Design review of the part built by this model. Coordinates are the model's own, in mm. A direction names the side the tool comes from. Give positions to 0.01 mm unless a question says otherwise; leave off trailing zeros. Order: outer loops, then holes, each group sorted by start corner. A loop starts at its lowest first (then second) coordinate and runs counter-clockwise, first axis right, second up.
Autodesk Inventor part; units mm, degrees
ref_plane "YZ Plane" through (0, 0, 0) normal (1, 0, 0) x (0, 1, 0)
ref_plane "XZ Plane" through (0, 0, 0) normal (0, 1, 0) x (-1, 0, 0)
ref_plane "XY Plane" through (0, 0, 0) normal (0, 0, 1) x (1, 0, 0)
sketch "Sketch1" plane through (0, 0, 0) normal (0, 0, 1) x (1, 0, 0)
  line L0 (36.9289, 8.8897) -> (11.5289, 8.8897)
  line L1 (36.9289, 148.5897) -> (36.9289, 8.8897)
  line L2 (11.5289, 148.5897) -> (36.9289, 148.5897)
  line L3 (20.8517, 15.2397) -> (20.8517, 142.2397)
  arc A0 (27.6081, 142.2397) -> (20.8517, 142.2397) centre (24.2299, 142.2397) ccw
  line L4 (27.6081, 142.2397) -> (27.6081, 15.2397)
  arc A1 (20.8517, 15.2397) -> (27.6081, 15.2397) centre (24.2299, 15.2397) ccw
  line L5 (36.9289, 148.5897) -> (11.5289, 148.5897)
  line L6 (11.5289, 148.5897) -> (11.5289, 8.8897)
  point P0 (0, 0)
  point P1 (0, 0)
  dimension "d0" = 25.4
  dimension "d2" = 139.7
  dimension "d5" = 6.35
  dimension "d6" = 6.35
  dimension "d7" = 3.3782
  dimension "d8" = 6.7564
  dimension "d9" = 3.3782
extrude "Plate1" add sketch "Sketch1" along normal blind 3.175
fillet "Corner Round1" radius 6.35 4 edges at (36.9289, 148.5897, 1.5875) (11.5289, 148.5897, 1.5875) (36.9289, 8.8897, 1.5875) (11.5289, 8.8897, 1.5875)
equation "\"BendRadius\" = Thickness"
equation "\"BendReliefWidth\" = Thickness"
equation "\"BendReliefDepth\" = 0.5 * Thickness"
equation "\"CornerReliefSize\" = 4 * Thickness"
equation "\"MinimumRemnant\" = 2 * Thickness"
equation "\"TransitionRadius\" = BendRadius"
equation "\"JacobiRadiusSize\" = BendRadius"
equation "\"GapSize\" = Thickness"
equation "\"d1\" = BendRadius"
properties part number "back brace mount" material "Aluminum 6061"
1. Machinability: for faces 4 (the face through (20.852, 78, 2)), 5 (the face through (35.02, 10.7, 1.61)), which of the approach directions +Z, -Z, +X, -X, +Y, -Y give a long, thin tool a straight path to every point of the face, cutting with its end or side? Answer none if there is none.
Recorded:
face 4: +Z, -Z
face 5: +Z, -Z, +X, -Y
2. Take a section at B-B (x = 25.5). State the section outline as (y, z) points (3 decimals), then the cut area to 3 significant figures.
Recorded:
outline: (8.89, 0) - (12.109, 0) - (12.109, 3.175) - (8.89, 3.175) - close; (145.37, 0) - (148.59, 0) - (148.59, 3.175) - (145.37, 3.175) - close
area: 20.4 mm2
3. Take a section at C-C (z = 2.5). State the section outline as (x, y) points, then the cut area to 3 significant figures.
Recorded:
outline: (11.53, 15.24) arc R6.35 ccw to (17.88, 8.89) - (30.58, 8.89) arc R6.35 ccw to (36.93, 15.24) - (36.93, 142.24) arc R6.35 ccw to (30.58, 148.59) - (17.88, 148.59) arc R6.35 ccw to (11.53, 142.24) - close; hole (20.85, 15.24) arc R3.38 ccw to (27.61, 15.24) - (27.61, 142.24) arc R3.38 ccw to (20.85, 142.24) - close
area: 2,620 mm2
4. Draft analysis for pull direction Y (two halves, no side actions). For faces 1 (the face through (30, 80, 3.175)), 2 (the face through (35.1, 146.7, 1.6)), 3 (the face through (24.304, 11.862, 1.565)), state which applies: pulls with the +Y half, pulls with the -Y half, needs draft (parallel to the pull), parting line crosses it, or undercut.
Recorded:
face 1: needs draft
face 2: pulls with the +Y half
face 3: undercut
5. For pin 1 (1 mm diameter, centred on x = 16.5, z = 1, fed in from +Y); pin 2 (2 mm diameter, centred on x = 23.5, y = 86, fed in from -Z), all flat-tipped, find the tip position at first contact; note any pin that passes through.
Recorded:
pin 1: stops at y = 148.53
pin 2: passes through
6. Take a section at A-A (y = 124.5). State the section outline as (x, z) points (3 decimals), then the cut area to 3 significant figures.
Recorded:
outline: (11.529, 0) - (20.852, 0) - (20.852, 3.175) - (11.529, 3.175) - close; (27.608, 0) - (36.929, 0) - (36.929, 3.175) - (27.608, 3.175) - close
area: 59.2 mm2
7. Take a section at D-D (x = 13.5). State the section outline as (y, z) points (3 decimals).
Recorded:
outline: (10.641, 0) - (146.838, 0) - (146.838, 3.175) - (10.641, 3.175) - close
8. For line 1 along X through (y, z) = (104.5, 1.6); line 2 along Y through (x, z) = (24, 2.2); line 3 along Y through (x, z) = (21.25, 2.3), list the stretches that pass through material, from the lowest coordinate up.
Recorded:
line 1: x = 11.53 to 20.85, 27.61 to 36.93
line 2: y = 8.89 to 11.87, 145.61 to 148.59
line 3: y = 8.89 to 13.65, 143.83 to 148.59
